The listing builds one solid part. Answer for the finished solid, in the listing's coordinates (mm). A direction names the side the tool comes from. Coordinates: 2 decimals unless noted, no trailing zeros. Order: outer loops, then holes, each group sorted by start corner. A loop starts at its lowest first (then second) coordinate and runs counter-clockwise, first axis right, second up. Notation, with made-up numbers: (5.25, 71) -> (30.25, 71) arc R18 ccw to (30.25, 83) -> close; hole circle Ø3 at (43.5, 67). An arc over 180 degrees is marked (long way). Answer in a Markdown table with one row per item. Add a question column.
```python
from build123d import *

# Parameters (mm, degrees)
SKETCH1_R                                      = 18.3
SKETCH1_R_2                                    = 4.65
INTEGRAL_HOLT_FLANGE_AND_STEM_CAVITY_DEPTH     = 23
SHARED_START                                   = 23
SKETCH2_R                                      = 22
SKETCH2_R_2                                    = 5.7
SKETCH2_R_3                                    = 2.3
SKETCH2_R_4                                    = 2.6
SHARED_FLAT_LOAD_PLATE_FOR_BOTH_CYLINDER_DEPTH = 4
LOWER_START                                    = 27
SKETCH3_W                                      = 66
SKETCH3_H                                      = 92.5
SKETCH3_R                                      = 22
SKETCH3_R_2                                    = 5.7
SKETCH3_R_3                                    = 2.3
LOWER_BEARING_AND_GUIDE_REGISTER_DEPTH         = 15


with BuildPart() as part:
    # Sketch1 → Integral HOLT flange and stem cavity (new body)
    with BuildSketch(Plane.XY):
        Polygon((-37, -43), (37, -43), (43, -37), (43, 37), (37, 43), (-37, 43), (-43, 37), (-43, -37), align=None)
        Circle(SKETCH1_R, mode=Mode.SUBTRACT)
        with Locations((-24.748737, -24.748737)):
            Circle(SKETCH1_R_2, mode=Mode.SUBTRACT)
        with Locations((-24.748737, 24.748737)):
            Circle(SKETCH1_R_2, mode=Mode.SUBTRACT)
        with Locations((24.748737, -24.748737)):
            Circle(SKETCH1_R_2, mode=Mode.SUBTRACT)
        with Locations((24.748737, 24.748737)):
            Circle(SKETCH1_R_2, mode=Mode.SUBTRACT)
    extrude(amount=INTEGRAL_HOLT_FLANGE_AND_STEM_CAVITY_DEPTH)

    # Sketch2 → Shared flat load plate for both cylinder mounts (add)
    with BuildSketch(Plane.XY.offset(SHARED_START)):
        Polygon((-96, -94), (96, -94), (104, -86), (104, 86), (96, 94), (-96, 94), (-104, 86), (-104, -86), align=None)
        Circle(SKETCH2_R, mode=Mode.SUBTRACT)
        with Locations((-24.748737, -24.748737)):
            Circle(SKETCH2_R_2, mode=Mode.SUBTRACT)
        with Locations((-24.748737, 24.748737)):
            Circle(SKETCH2_R_2, mode=Mode.SUBTRACT)
        with Locations((24.748737, -24.748737)):
            Circle(SKETCH2_R_2, mode=Mode.SUBTRACT)
        with Locations((24.748737, 24.748737)):
            Circle(SKETCH2_R_2, mode=Mode.SUBTRACT)
        with Locations((-96, -88)):
            Circle(SKETCH2_R_3, mode=Mode.SUBTRACT)
        with Locations((-96, 88)):
            Circle(SKETCH2_R_3, mode=Mode.SUBTRACT)
        with Locations((96, -88)):
            Circle(SKETCH2_R_3, mode=Mode.SUBTRACT)
        with Locations((96, 88)):
            Circle(SKETCH2_R_3, mode=Mode.SUBTRACT)
        with Locations((34.5, 60)):
            Circle(SKETCH2_R_4, mode=Mode.SUBTRACT)
        with Locations((34.5, 78)):
            Circle(SKETCH2_R_4, mode=Mode.SUBTRACT)
        with Locations((-34.5, -60)):
            Circle(SKETCH2_R_4, mode=Mode.SUBTRACT)
        with Locations((-34.5, -78)):
            Circle(SKETCH2_R_4, mode=Mode.SUBTRACT)
    extrude(amount=SHARED_FLAT_LOAD_PLATE_FOR_BOTH_CYLINDER_DEPTH)

    # Sketch3 → Lower bearing and guide register (add)
    with BuildSketch(Plane.XY.offset(LOWER_START)):
        Rectangle(SKETCH3_W, SKETCH3_H)
        Circle(SKETCH3_R, mode=Mode.SUBTRACT)
        with Locations((-24.748737, -24.748737)):
            Circle(SKETCH3_R_2, mode=Mode.SUBTRACT)
        with Locations((-24.748737, 24.748737)):
            Circle(SKETCH3_R_2, mode=Mode.SUBTRACT)
        with Locations((24.748737, -24.748737)):
            Circle(SKETCH3_R_2, mode=Mode.SUBTRACT)
        with Locations((24.748737, 24.748737)):
            Circle(SKETCH3_R_2, mode=Mode.SUBTRACT)
        with Locations((-28, -40.5)):
            Circle(SKETCH3_R_3, mode=Mode.SUBTRACT)
        with Locations((-28, 40.5)):
            Circle(SKETCH3_R_3, mode=Mode.SUBTRACT)
        with Locations((28, -40.5)):
            Circle(SKETCH3_R_3, mode=Mode.SUBTRACT)
        with Locations((28, 40.5)):
            Circle(SKETCH3_R_3, mode=Mode.SUBTRACT)
    extrude(amount=LOWER_BEARING_AND_GUIDE_REGISTER_DEPTH)


solid = part.part
```
Q1. A cutting plane is placed at B-B (y = -60). Determine the outline of the cut face in (x, z), then the cut area to 3 significant figures.
Q2. Straight lines are drawn through the part: line 1 (Y direction, x = 96, z = 25.95); line 2 (Y direction, x = 0, z = 18); line 3 (Y direction, x = -34, z = 25). For each, find the intervals that lie inside material, in ascending order.
Q3. For faces 5 (the face through (-100, -90, 25)), 6 (the face through (-28, 41, 27)), 7 (the face through (40, 40, 11)), 8 (the face through (33, -1, 34)), determine the directions among +Z, -Z, +X, -X, +Y, -Y from which every point of the face is accessible in a straight line to the end or side of a thin tool.
Q4. Given pin 1 (7.5 mm diameter, centred on x = 1, z = 36.5, fed in from -Y); pin 2 (7 mm diameter, centred on y = 0, z = 6.5, fed in from -X); pin 3 (4.5 mm diameter, centred on y = 8, z = 36.5, fed in from -X), each flat-ended and moving along its own axis, determine where each tip first touches the part or whether it passes through.
Q5. Determine the mould class of faces 1 (the face through (-40, -40, 11)), 2 (the face through (1, 43, 11)), 3 (the face through (-29.825, 39.1, 34.395)), 4 (the face through (28, 41, 27)) for opening direction X: +X half, -X half, draft (parallel to the pull), parting line (faces both ways), or undercut.
Q6. A cutting plane is placed at A-A (x = 0). Determine the outline of the cut face in (y, z).
Q7. A cutting plane is placed at C-C (y = -40.5). Determine the outline of the cut face in (x, z).
Q8. A cutting plane is placed at D-D (z = 13.5). Determine the outline of the cut face in (x, y).
Returned:
| question | item | result |
|---|---|---|
| 1 | outline | (-104, 23) -> (-37.1, 23) -> (-37.1, 27) -> (-104, 27) -> close; (-31.9, 23) -> (104, 23) -> (104, 27) -> (-31.9, 27) -> close |
| 1 | area | 811 mm² |
| 2 | line 1 | y = -94 to -90.3, -85.7 to 85.7, 90.3 to 94 |
| 2 | line 2 | y = -43 to -18.3, 18.3 to 43 |
| 2 | line 3 | y = -94 to -80.55, -75.45 to -62.55, -57.45 to 94 |
| 3 | face 5 | +Z, -Z, -X, -Y |
| 3 | face 6 | +Z |
| 3 | face 7 | -Z, +X, +Y |
| 3 | face 8 | +Z, +X, +Y, -Y |
| 4 | pin 1 | stops at y = -46.25 |
| 4 | pin 2 | stops at x = -43 |
| 4 | pin 3 | stops at x = -33 |
| 5 | face 1 | -X half |
| 5 | face 2 | draft |
| 5 | face 3 | undercut |
| 5 | face 4 | undercut |
| 6 | outline | (-94, 23) -> (-43, 23) -> (-43, 0) -> (-18.3, 0) -> (-18.3, 23) -> (-22, 23) -> (-22, 42) -> (-46.25, 42) -> (-46.25, 27) -> (-94, 27) -> close; (18.3, 0) -> (43, 0) -> (43, 23) -> (94, 23) -> (94, 27) -> (46.25, 27) -> (46.25, 42) -> (22, 42) -> (22, 23) -> (18.3, 23) -> close |
| 7 | outline | (-104, 23) -> (-39.5, 23) -> (-39.5, 0) -> (39.5, 0) -> (39.5, 23) -> (104, 23) -> (104, 27) -> (33, 27) -> (33, 42) -> (30.3, 42) -> (30.3, 27) -> (25.7, 27) -> (25.7, 42) -> (-25.7, 42) -> (-25.7, 27) -> (-30.3, 27) -> (-30.3, 42) -> (-33, 42) -> (-33, 27) -> (-104, 27) -> close |
| 8 | outline | (-43, -37) -> (-37, -43) -> (37, -43) -> (43, -37) -> (43, 37) -> (37, 43) -> (-37, 43) -> (-43, 37) -> close; hole circle Ø9.3 at (-24.75, -24.75); hole circle Ø9.3 at (-24.75, 24.75); hole circle Ø36.6 at (0, 0); hole circle Ø9.3 at (24.75, -24.75); hole circle Ø9.3 at (24.75, 24.75) |
